Geometry: see drawing. Coordinates: mm, zero at the bounding-box minimum. A direction names the side the tool comes from. Give positions to 0.01 mm unless a question says otherwise; leave off trailing zeros. Write each loop counter-clockwise with the first axis right and the second up, starting at its lowest first coordinate (ties: lowest second). Pieces come first, ordered by that corner, then holes. Notation, with made-up numbers: (1, -37) - (10, -37) arc R24 ccw to (10, -20) - close; hole circle Ø9 at (42, -13.5). An arc over 180 degrees is marked (long way). Answer as CSV lines item,"result". Start each with the question number.
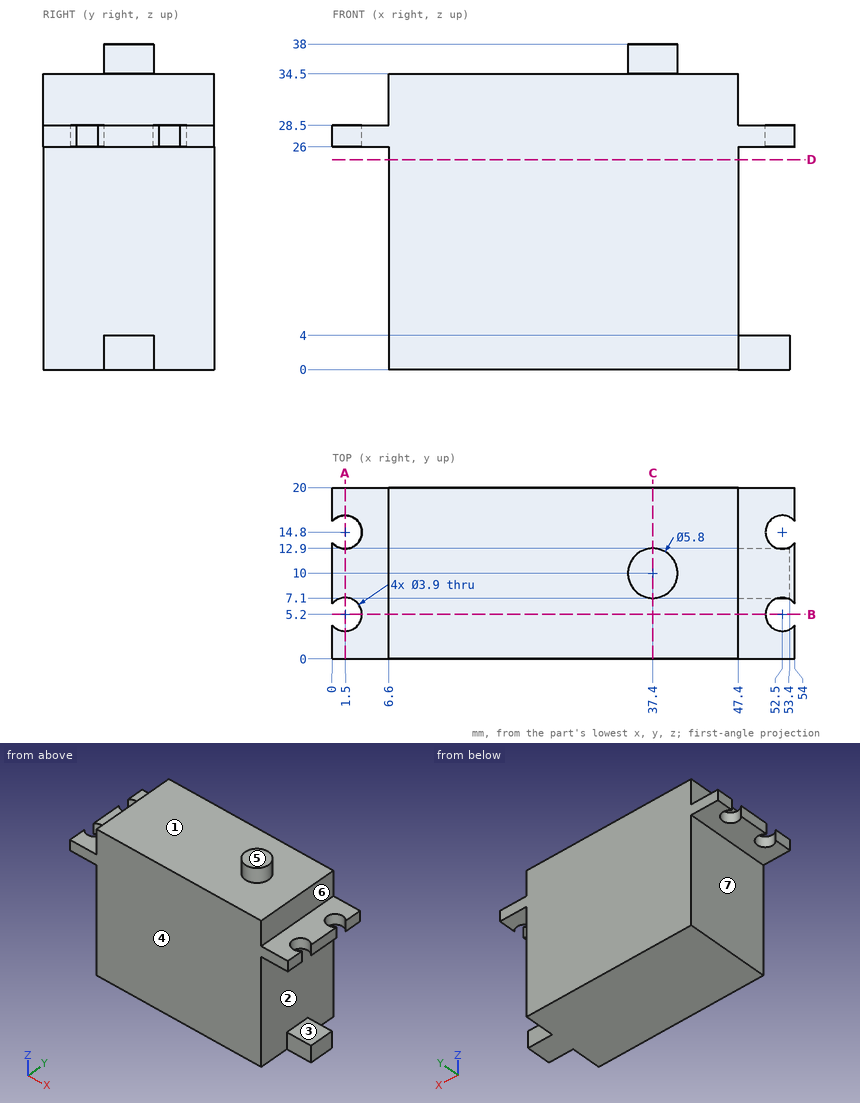
1) Contact query for flat-ended pins moving along their axis: P1, Ø12, axis at y = 15, z = 7, coming from the +X side; P2, Ø6, axis at y = 8, z = 22, coming from the +X side; P3, Ø2, axis at x = 2, y = 9, coming from the +Z side. Output: stop coordinate, or through.
2) Cut plane D-D on z = 24.5. Output: boundary loops of the cut face in (x, y), and give its area (3 significant figures).
3) Material intervals for line 1 (Y direction, x = 1.5, z = 26.9); line 2 (Z direction, x = 19, y = 15.5); line 3 (X direction, y = 11, z = 20), sorted ascending. Write a range as from..to.
4) Pull-direction query (Z, two-part tool) for the marked faces 1, 2, 3 and 4; classes: +Z half, -Z half, draft (parallel to the pull), parting line (faces both ways), or undercut.
5) Cut plane A-A on x = 1.5. Output: boundary loops of the cut face in (y, z).
6) Reachability of the marked faces 5, 6 and 7 from +Z, -Z, +X, -X, +Y, -Y: full face, straight path, thin tool, end or side. Return the list, or none.
7) Cut plane B-B on y = 5.2. Output: boundary loops of the cut face in (x, z), and give its area (3 significant figures).
8) Cut plane C-C on x = 37.4. Output: boundary loops of the cut face in (y, z), and give its area (3 significant figures).
Numbers:
1,P1,"stops at x = 53.4"
1,P2,"stops at x = 47.4"
1,P3,"stops at z = 28.5"
2,outline,"(6.6, 0) - (47.4, 0) - (47.4, 20) - (6.6, 20) - close"
2,area,"816 mm²"
3,line 1,"y = 0..3.25, 7.15..12.85, 16.75..20"
3,line 2,"z = 0..34.5"
3,line 3,"x = 6.6..47.4"
4,face 1,"+Z half"
4,face 2,"undercut"
4,face 3,"undercut"
4,face 4,"draft"
5,outline,"(0, 26) - (3.25, 26) - (3.25, 28.5) - (0, 28.5) - close; (7.15, 26) - (12.85, 26) - (12.85, 28.5) - (7.15, 28.5) - close; (16.75, 26) - (20, 26) - (20, 28.5) - (16.75, 28.5) - close"
6,face 5,"+Z, +X, -X, +Y, -Y"
6,face 6,"+Z, +X, +Y, -Y"
6,face 7,"-Z, -X, +Y, -Y"
7,outline,"(3.45, 26) - (6.6, 26) - (6.6, 0) - (47.4, 0) - (47.4, 26) - (50.55, 26) - (50.55, 28.5) - (47.4, 28.5) - (47.4, 34.5) - (6.6, 34.5) - (6.6, 28.5) - (3.45, 28.5) - close"
7,area,"1,420 mm²"
8,outline,"(0, 0) - (20, 0) - (20, 34.5) - (12.9, 34.5) - (12.9, 38) - (7.1, 38) - (7.1, 34.5) - (0, 34.5) - close"
8,area,"710 mm²"
